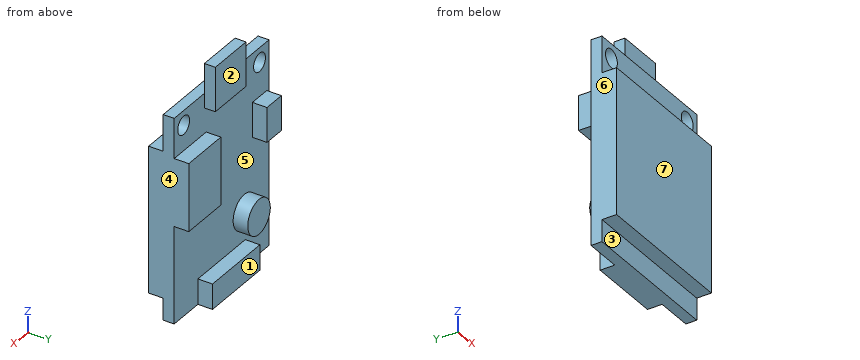
Autodesk Inventor part; units mm, degrees
ref_plane "YZ Plane" through (0, 0, 0) normal (1, 0, 0) x (0, 1, 0)
ref_plane "XZ Plane" through (0, 0, 0) normal (0, 1, 0) x (-1, 0, 0)
ref_plane "XY Plane" through (0, 0, 0) normal (0, 0, 1) x (1, 0, 0)
sketch "Sketch1" plane through (0, 0, 0) normal (0, 1, 0) x (-1, 0, 0)
  line L0 (0, 0) -> (20, 0)
  line L1 (20, 0) -> (20, -28)
  line L2 (20, -28) -> (0, -28)
  line L3 (0, -28) -> (0, 0)
  dimension "d0" = 28
  dimension "d1" = 20
extrude "Extrusion1" add sketch "Sketch1" along normal blind 1.5
sketch "Sketch2" plane through (0, 1.5, 0) normal (0, 1, 0) x (1, 0, 0)
  line L0 (0, 28) -> (-20, 28)
  line L1 (-5, 28) -> (-15, 28)
  line L2 (-15, 28) -> (-15, 24.5354)
  line L3 (-15, 24.5354) -> (-5, 24.5354)
  line L4 (-5, 24.5354) -> (-5, 28)
  point P0 (0, 0)
  point P1 (-10, 24.5354)
  point P2 (-10, 28)
  dimension "d4" = 10
extrude "Extrusion2" add sketch "Sketch2" along normal blind 2
sketch "Sketch3" plane through (0, 1.5, 0) normal (0, 1, 0) x (1, 0, 0)
  line L0 (0, 0) -> (0, 28)
  line L1 (0, 5.4716) -> (-6.7562, 5.4716)
  line L2 (-6.7562, 5.4716) -> (-6.7562, 14.73)
  line L3 (-6.7562, 14.73) -> (0, 14.73)
  line L4 (0, 14.73) -> (0, 5.4716)
extrude "Extrusion3" add sketch "Sketch3" along normal blind 2
sketch "Sketch4" plane through (0, 1.5, 0) normal (0, 1, 0) x (1, 0, 0)
  circle A0 centre (-14.8135, 20.6337) radius 2.3748
  point P0 (0, 0)
extrude "Extrusion4" add sketch "Sketch4" along normal blind 2
sketch "Sketch5" plane through (0, 1.5, 0) normal (0, 1, 0) x (1, 0, 0)
  circle A0 centre (-2, 2) radius 1.25
  circle A1 centre (-18, 2) radius 1.25
  line L0 (0, 0) -> (0, 5.4716)
  line L1 (-20, 0) -> (0, 0)
  line L2 (-20, 28) -> (-20, 0)
  dimension "d11" = 2
  dimension "d12" = 2.5
  dimension "d13" = 2
  dimension "d14" = 2
  dimension "d15" = 2
  dimension "d16" = 2.5
extrude "Extrusion5" cut sketch "Sketch5" against normal blind 2
sketch "Sketch6" plane through (0, 0, 0) normal (0, -1, 0) x (1, 0, 0)
  line L0 (-20, 0) -> (-20, -28)
  line L1 (-20, -25) -> (0, -25)
  line L2 (0, -25) -> (0, -5)
  line L3 (0, -5) -> (-20, -5)
  line L4 (-20, -5) -> (-20, -25)
  line L5 (-20, -28) -> (0, -28)
  line L6 (0, 0) -> (-20, 0)
  dimension "d19" = 3
  dimension "d20" = 5
extrude "Extrusion6" add sketch "Sketch6" along normal blind 2
sketch "Sketch7" plane through (0, 1.5, 0) normal (0, 1, 0) x (1, 0, 0)
  line L0 (-16.4979, 6.6511) -> (-19.5294, 6.6511)
  line L1 (-19.5294, 6.6511) -> (-19.5294, 11.4005)
  line L2 (-19.5294, 11.4005) -> (-16.4979, 11.4005)
  line L3 (-16.4979, 11.4005) -> (-16.4979, 6.6511)
  point P0 (0, 0)
extrude "Extrusion7" add sketch "Sketch7" along normal blind 2
sketch "Sketch8" plane through (0, 1.5, 0) normal (0, 1, 0) x (1, 0, 0)
  line L0 (-12.8387, 1.9896) -> (-6.3724, 1.9896)
  line L1 (-6.3724, 1.9896) -> (-6.3724, -4.0656)
  line L2 (-6.3724, -4.0656) -> (-12.8387, -4.0656)
  line L3 (-12.8387, -4.0656) -> (-12.8387, 1.9896)
  point P0 (0, 0)
extrude "Extrusion8" add sketch "Sketch8" along normal blind 1.5
equation "\"d16\" = d12"
properties part number "VideoTransmitter" material "ABS Plastic"
Could you check a few things on this model? Use its own coordinates, in mm. Face numbers are marked on the shaded views. A direction names the side the tool comes from. Give positions to 0.01 mm unless a question says otherwise; leave off trailing zeros. Order: outer loops, then holes, each group sorted by start corner. A loop starts at its lowest first (then second) coordinate and runs counter-clockwise, first axis right, second up. Notation, with made-up numbers: (-38.5, 45.5) -> (-22.5, 45.5) arc R15 cw to (-22.5, 71.5) -> close; hole circle Ø9 at (66.25, -36). An arc over 180 degrees is marked (long way). Return JSON: item names as keys, results as strings.
1. I need wall thicknesses on line 1 (X direction, y = 0.4, z = -2); line 2 (X direction, y = 3.1, z = -11); line 3 (Z direction, x = -18, y = 0.8). Which ranges of each line are inside material? Lowest first, please. Write a range as from..to.
Answer list:
{"line 1": "x = -20..-19.25, -16.75..-3.25, -0.75..0", "line 2": "x = -19.53..-16.5, -6.76..0", "line 3": "z = -28..-3.25, -0.75..0"}
2. On a 3-axis mill with a long thin cutter (end or side, diameter ignored), from which of +Z, -Z, +X, -X, +Y, -Y can I reach the whole of each face in a straight line? I mean the marked faces 1, 2 and 3. Say none if no direction works.
Answer list:
{"face 1": "+Z, -Z, +X, -X, +Y", "face 2": "+Z, +X, -X, +Y", "face 3": "-Z, +X, -X, -Y"}
3. Imagine slicing it at B-B on y = 0.35. List the corners of the cut face in (x, z) for me.
Answer list:
{"outline": "(-20, -28) -> (0, -28) -> (0, 0) -> (-20, 0) -> close; hole circle Ø2.5 at (-18, -2); hole circle Ø2.5 at (-2, -2)"}
4. For pin 1 Ø2 at (x, y) = (-4.5, 2) entering from +Z; pin 2 Ø1.2 at (x, z) = (-11, 1.5) entering from -Y; pin 3 Ø1 at (y, z) = (2.5, -12) entering from -X; pin 4 Ø2 at (x, z) = (-18, -2) entering from +Y, each with a flat end and sliding along its axis, tell me the tip position at first contact or that it passes through.
Answer list:
{"pin 1": "stops at z = 0", "pin 2": "stops at y = 1.5", "pin 3": "stops at x = -6.76", "pin 4": "passes through"}
5. Imagine slicing it at A-A on x = -18. List the corners of the cut face in (y, z) for me, then the cut area to 3 significant figures.
Answer list:
{"outline": "(-2, -25) -> (0, -25) -> (0, -28) -> (1.5, -28) -> (1.5, -11.4) -> (3.5, -11.4) -> (3.5, -6.65) -> (1.5, -6.65) -> (1.5, -3.25) -> (0, -3.25) -> (0, -5) -> (-2, -5) -> close; (0, -0.75) -> (1.5, -0.75) -> (1.5, 0) -> (0, 0) -> close", "area": "87.7 mm2"}
6. Imagine slicing it at C-C on x = -2. List the corners of the cut face in (y, z) for me, then the cut area to 3 significant figures.
Answer list:
{"outline": "(-2, -25) -> (0, -25) -> (0, -28) -> (1.5, -28) -> (1.5, -14.73) -> (3.5, -14.73) -> (3.5, -5.47) -> (1.5, -5.47) -> (1.5, -3.25) -> (0, -3.25) -> (0, -5) -> (-2, -5) -> close; (0, -0.75) -> (1.5, -0.75) -> (1.5, 0) -> (0, 0) -> close", "area": "96.8 mm2"}
7. Thinking about a two-plate mould opening in X: for the marked faces 4, 5, 6 and 7, which applies, pulls with the +X half, pulls with the -X half, needs draft (parallel to the pull), parting line crosses it, or undercut?
Answer list:
{"face 4": "pulls with the +X half", "face 5": "undercut", "face 6": "pulls with the -X half", "face 7": "needs draft"}
8. Imagine slicing it at D-D on z = 2. List the corners of the cut face in (x, y) for me.
Answer list:
{"outline": "(-12.84, 1.5) -> (-6.37, 1.5) -> (-6.37, 3) -> (-12.84, 3) -> close"}
